Check sheet for the modelled part. Datum: model origin and axes. Units: mm. Face numbers are marked on the shaded views. A direction names the side the tool comes from. Give positions to 0.01 mm unless a question says otherwise; leave off trailing zeros. Write each loop counter-clockwise with the first axis right and the second up, starting at its lowest first coordinate (ties: lowest second). Pieces come first, ordered by that corner, then holes.
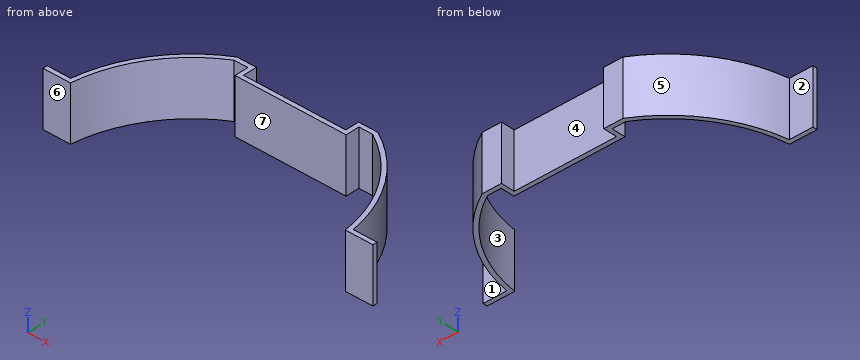
from build123d import *

# Parameters (mm, degrees)
F1_DEPTH = 25.4


# Not quite as in the source:
# - a pattern or mirror of a feature is missing from the dataset's text; its kind, count and spacing are read off the source's solid


with BuildPart() as f1:
    # F0 (on Top) → F1 (new body)
    with BuildSketch(Plane.XY):
        with BuildLine():
            Line((-25.654, 0), (0, 0))
            Line((0, 0), (0, 2.032))
            Line((0, 2.032), (-23.622, 2.032))
            Line((-23.622, 2.032), (-23.622, 8.382))
            Line((-23.622, 8.382), (-32.5398903871, 8.382))
            ThreePointArc((-32.5398903871, 8.382), (-54.4156625214, -11.5711123989), (-65.2763838561, -39.116))
            Line((-65.2763838561, -39.116), (-76.2, -39.116))
            Line((-76.2, -39.116), (-76.2, -41.148))
            Line((-76.2, -41.148), (-63.5, -41.148))
            ThreePointArc((-63.5, -41.148), (-53.3799799525, -13.6670774646), (-32.004, 6.35))
            Line((-32.004, 6.35), (-25.654, 6.35))
            Line((-25.654, 6.35), (-25.654, 0))
        make_face()
    extrude(amount=F1_DEPTH)

    # F1_copies: F1 across plane


with BuildPart() as f1_1:
    add(f1.part)
    add(f1.part.mirror(Plane(origin=(0, 0, 0), x_dir=(0, 0, 1), z_dir=(1, 0, 0))))


solid = f1_1.part
1) Scan lines: L1, parallel to X at y = -18.5, z = 10.75; L2, parallel to X at y = 5, z = 9.75; L3, parallel to Y at x = -12, z = 2. Record each from-to range of solid material in increasing order.
2) Sectioned sample at A-A on y = -36. Record the boundary of the cut face in (x, z).
3) Sectioned sample at B-B on z = 21. Record the boundary of the cut face in (x, y), then the cut area to 3 significant figures.
4) Sectioned sample at D-D on y = -19. Record the boundary of the cut face in (x, z).
5) Gauge pin test, flat ends, axial feed: pin 1 (5 mm diameter, centred on x = -1.5, z = 12, fed in from -Y); pin 2 (1.9 mm diameter, centred on y = 5, z = 11.5, fed in from -X); pin 3 (12.5 mm diameter, centred on x = 0, z = 14.5, fed in from +Y). Record the tip position at first contact, or that the pin passes through.
6) Sectioned sample at C-C on x = -13. Record the boundary of the cut face in (y, z), then the cut area to 3 significant figures.
7) Access from +Z, -Z, +X, -X, +Y, -Y to the whole of each face (thin tool, end or side, straight path). Record for the marked faces 1, 2, 3 and 4.
8) Draft check along X on the marked faces 5, 6 and 7. Enter one of: +X half, -X half, draft (parallel to the pull), parting line (faces both ways), or undercut.
Answers below:
1. L1: x = -58.59 to -56.28, 56.28 to 58.59
1. L2: x = -37.93 to -34.25, -25.65 to -23.62, 23.62 to 25.65, 34.25 to 37.93
1. L3: y = 0 to 2.03
2. outline: (-64.74, 0) - (-62.66, 0) - (-62.66, 25.4) - (-64.74, 25.4) - close; (62.66, 0) - (64.74, 0) - (64.74, 25.4) - (62.66, 25.4) - close
3. outline: (-76.2, -41.15) - (-63.5, -41.15) arc R63.5 cw to (-32, 6.35) - (-25.65, 6.35) - (-25.65, 0) - (25.65, 0) - (25.65, 6.35) - (32, 6.35) arc R63.5 cw to (63.5, -41.15) - (76.2, -41.15) - (76.2, -39.12) - (65.28, -39.12) arc R65.53 ccw to (32.54, 8.38) - (23.62, 8.38) - (23.62, 2.03) - (-23.62, 2.03) - (-23.62, 8.38) - (-32.54, 8.38) arc R65.53 ccw to (-65.28, -39.12) - (-76.2, -39.12) - close
3. area: 446 mm2
4. outline: (-58.84, 0) - (-56.55, 0) - (-56.55, 25.4) - (-58.84, 25.4) - close; (56.55, 0) - (58.84, 0) - (58.84, 25.4) - (56.55, 25.4) - close
5. pin 1: stops at y = 0
5. pin 2: stops at x = -39.26
5. pin 3: stops at y = 2.03
6. outline: (0, 0) - (2.03, 0) - (2.03, 25.4) - (0, 25.4) - close
6. area: 51.6 mm2
7. face 1: +Z, -Z, +X, +Y
7. face 2: +Z, -Z, -X, +Y
7. face 3: +Z, -Z, -Y
7. face 4: +Z, -Z, +Y
8. face 5: -X half
8. face 6: draft
8. face 7: undercut
